```python
from build123d import *

# Parameters (mm, degrees)
SFAZOWANIE1_SIZE = 1
SFAZOWANIE2_SIZE = 1


with BuildPart() as part:
    # Szkic1 → Obrót1 (revolve)
    with BuildSketch(Plane(origin=(0, 0, 0), x_dir=(0, 0, -1), z_dir=(1, 0, 0)), mode=Mode.PRIVATE) as obr_t1_sk:
        Polygon((0, 0), (600, 0), (600, 6), (584, 6), (584, 8), (52, 8), (52, 6), (22, 6), (22, 5), (9, 5), (9, 4), (0, 4), align=None)
    revolve(obr_t1_sk.sketch.rotate(Axis((0, 0, 0), (0, 0, -1)), 90), axis=Axis((0, 0, 0), (0, 0, -1)))

    # Sfazowanie1
    sfazowanie1_edges = [part.edges().sort_by_distance(p)[0] for p in [
        (-6, 0, -22),
        (-4, 0, 0),
        (-5, 0, -9),
    ]]
    chamfer(sfazowanie1_edges, length=SFAZOWANIE1_SIZE - 0.0001)  # a hair under: the kernel refuses the full size

    # Sfazowanie2
    sfazowanie2_edges = [part.edges().sort_by_distance(p)[0] for p in [
        (-6, 0, -600),
    ]]
    chamfer(sfazowanie2_edges, length=SFAZOWANIE2_SIZE)


solid = part.part
```
Could you check a few things on this model? Use its own coordinates, in mm. A direction names the side the tool comes from. Round coordinates to 2 decimals unless told otherwise and drop trailing zeros. Loops run counter-clockwise (first coordinate to the right, second up) from the corner with the lowest first, then second, coordinate; pieces in that order, holes last. Notation, with made-up numbers: (-17.75, 42) - (15.25, 42) arc R30 cw to (15.25, 77) - close; hole circle Ø3 at (68.25, 25). An arc over 180 degrees is marked (long way). Answer in a Markdown table with one row per item. Add a question column.
(1) If we section it at C-C (z = -116): Please give me the cut outline in (x, y).
(2) For faces 1 (the face through (-1.73, 7.81, -314.28)), 2 (the face through (2, -6, -584)), 3 (the face through (-5, 0, -16)), which set-ups out of +Z, -Z, +X, -X, +Y, -Y let a thin tool reach every point of the face, with its end or its side?
(3) I need wall thicknesses on line 1 along Y through (x, z) = (1, -520.5); line 2 along X through (y, z) = (-1.25, -445.5); line 3 along Y through (x, z) = (-0.25, -259). Which ranges of each line are inside material? Lowest first, please.
(4) I'm going to push flat-ended pins straight in: pin 1 (1 mm diameter, centred on x = -2, z = -241.5, fed in from +Y); pin 2 (1.5 mm diameter, centred on x = 1, y = -6, fed in from -Z); pin 3 (4 mm diameter, centred on y = 4, z = -248, fed in from -X). Where does each tip first touch, or does it pass through?
Model answer:
| question | item | result |
|---|---|---|
| 1 | outline | circle Ø16 at (0, 0) |
| 2 | face 1 | +Z, -Z |
| 2 | face 2 | -Z |
| 2 | face 3 | +Z |
| 3 | line 1 | y = -7.94 to 7.94 |
| 3 | line 2 | x = -7.9 to 7.9 |
| 3 | line 3 | y = -8 to 8 |
| 4 | pin 1 | stops at y = 7.86 |
| 4 | pin 2 | stops at z = -599.67 |
| 4 | pin 3 | stops at x = -7.75 |
